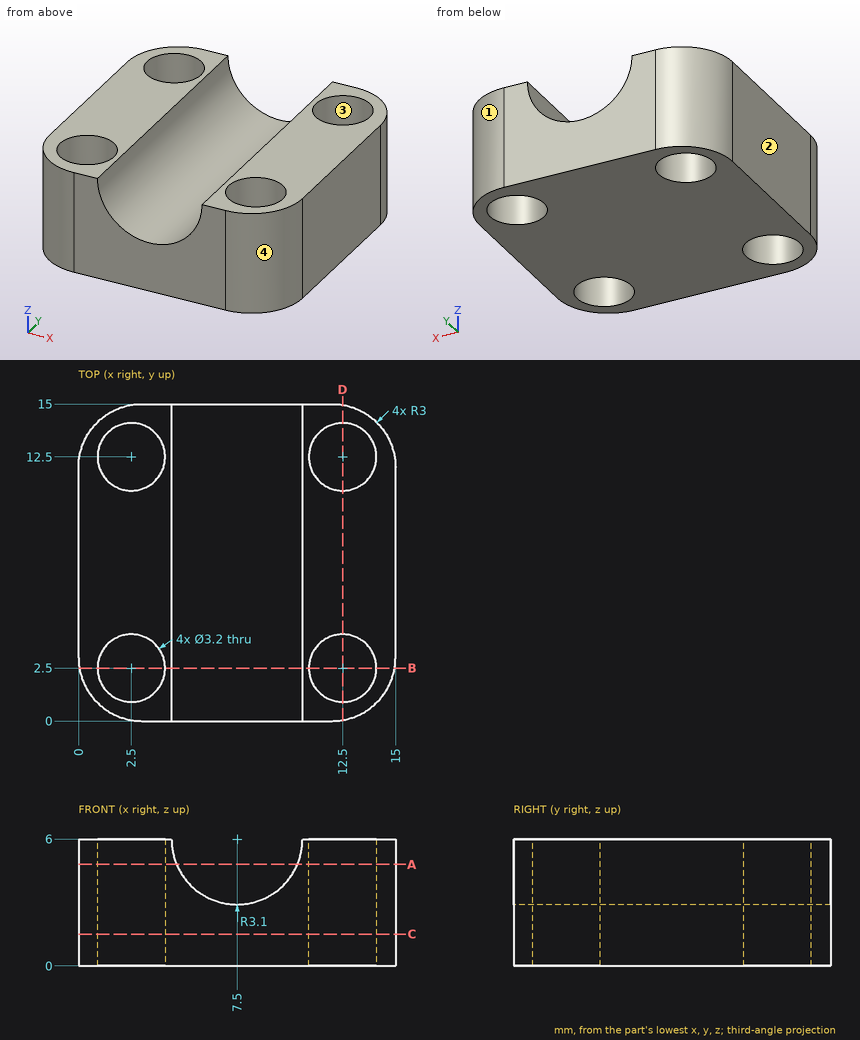
Verification items for this drawing (mm, ordinates from the low corner). Coordinates: 2 decimals unless noted, no trailing zeros. Write each loop counter-clockwise with the first axis right and the second up, starting at its lowest first coordinate (ties: lowest second). Pieces come first, ordered by that corner, then holes. Notation, with made-up numbers: M -13.75,9 L 23.25,9 A19 cw 23.25,40 Z; hole C 52.25,32 d8. An arc over 180 degrees is marked long. Use one line per item in the form item = value. Start each with the question number.
1) Section check B-B on y = 2.5. Enter the section's corners in (x, z), and give its area (3 significant figures).
2) Go/stop test with flat-tipped pins: pin 1 Ø2.5 at (x, y) = (12.5, 2.5) entering from +Z; pin 2 Ø1 at (x, z) = (13.5, 3) entering from +Y. Record where each tip stops, or that it passes through.
3) Section check A-A on z = 4.8. Enter the section's corners in (x, y).
4) Thickness scan on probe 1 along Y at (x, z) = (12.5, 3.55); probe 2 along Y at (x, z) = (13.25, 3.2); probe 3 along X at (y, z) = (12, 3.4). Record the ranges inside material, lowest first. Write a range as from..to.
5) Section check D-D on x = 12.5. Enter the section's corners in (y, z), and give its area (3 significant figures).
6) Release check for a two-part mould opening along Y. For the marked faces 1, 2, 3 and 4 record: pulls with the +Y half, pulls with the -Y half, needs draft (parallel to the pull), parting line crosses it, or undercut.
7) Section check C-C on z = 1.5. Enter the section's corners in (x, y), and give its area (3 significant figures).
Responses:
q1.outline = M 0.04,0 L 0.9,0 L 0.9,6 L 0.04,6 Z; M 4.1,0 L 10.9,0 L 10.9,6 L 10.6,6 A3.1 cw 4.4,6 L 4.1,6 Z; M 14.1,0 L 14.96,0 L 14.96,6 L 14.1,6 Z
q1.area = 36.0 mm2
q2.pin_1 = through
q2.pin_2 = 14.83
q3.outline = M 0,3 A3 ccw 3,0 L 4.64,0 L 4.64,15 L 3,15 A3 ccw 0,12 Z; M 10.36,0 L 12,0 A3 ccw 15,3 L 15,12 A3 ccw 12,15 L 10.36,15 Z; hole C 2.5,2.5 d3.2; hole C 2.5,12.5 d3.2; hole C 12.5,2.5 d3.2; hole C 12.5,12.5 d3.2
q4.probe_1 = 0.04..0.9, 4.1..10.9, 14.1..14.96
q4.probe_2 = 0.27..1.09, 3.91..11.09, 13.91..14.73
q4.probe_3 = 0..0.98, 4.02..5.81, 9.19..10.98, 14.02..15
q5.outline = M 0.04,0 L 0.9,0 L 0.9,6 L 0.04,6 Z; M 4.1,0 L 10.9,0 L 10.9,6 L 4.1,6 Z; M 14.1,0 L 14.96,0 L 14.96,6 L 14.1,6 Z
q5.area = 51.1 mm2
q6.face_1 = pulls with the +Y half
q6.face_2 = needs draft
q6.face_3 = undercut
q6.face_4 = pulls with the -Y half
q7.outline = M 0,3 A3 ccw 3,0 L 12,0 A3 ccw 15,3 L 15,12 A3 ccw 12,15 L 3,15 A3 ccw 0,12 Z; hole C 2.5,2.5 d3.2; hole C 2.5,12.5 d3.2; hole C 12.5,2.5 d3.2; hole C 12.5,12.5 d3.2
q7.area = 185 mm2
